```python
from build123d import *

# Parameters (mm, degrees)
CYLINDER009_R     = 0.8
CYLINDER009_DEPTH = 20
CYLINDER010_R     = 0.8
CYLINDER010_DEPTH = 20
CYLINDER011_R     = 0.8
CYLINDER011_DEPTH = 20
CYLINDER008_R     = 0.8
CYLINDER008_DEPTH = 20
CYLINDER005_R     = 0.34
CYLINDER005_DEPTH = 100
CYLINDER006_R     = 0.34
CYLINDER006_DEPTH = 100
CYLINDER007_R     = 0.34
CYLINDER007_DEPTH = 100
CYLINDER004_R     = 0.34
CYLINDER004_DEPTH = 100
CYLINDER002_R     = 4.6
CYLINDER002_DEPTH = 0.5
CYLINDER003_R     = 4.6
CYLINDER003_DEPTH = 0.5
BOX008_W          = 18
BOX008_H          = 9.2
BOX008_DEPTH      = 0.5
BOX004_W          = 40
BOX004_H          = 1
BOX004_DEPTH      = 2.5
CYLINDER001_R     = 2
CYLINDER001_DEPTH = 20
BOX002_W          = 40
BOX002_H          = 42
BOX002_DEPTH      = 6
BOX001_W          = 42
BOX001_H          = 44
BOX001_DEPTH      = 7
BOX003_W          = 40
BOX003_H          = 1
BOX003_DEPTH      = 2.5


with BuildPart() as zylinder009:
    # Cylinder009 → Cylinder009 (new body)
    with BuildSketch(Plane(origin=(2.5, 2.5, -10), x_dir=(1, 0, 0), z_dir=(0, 0, 1))):
        Circle(CYLINDER009_R)
    extrude(amount=CYLINDER009_DEPTH)


with BuildPart() as zylinder010:
    # Cylinder010 → Cylinder010 (new body)
    with BuildSketch(Plane(origin=(37.5, 39.5, -10), x_dir=(1, 0, 0), z_dir=(0, 0, 1))):
        Circle(CYLINDER010_R)
    extrude(amount=CYLINDER010_DEPTH)


with BuildPart() as zylinder011:
    # Cylinder011 → Cylinder011 (new body)
    with BuildSketch(Plane(origin=(2.5, 39.5, -10), x_dir=(1, 0, 0), z_dir=(0, 0, 1))):
        Circle(CYLINDER011_R)
    extrude(amount=CYLINDER011_DEPTH)


with BuildPart() as compound005:
    # Cylinder008 → Cylinder008 (new body)
    with BuildSketch(Plane(origin=(37.5, 2.5, -10), x_dir=(1, 0, 0), z_dir=(0, 0, 1))):
        Circle(CYLINDER008_R)
    extrude(amount=CYLINDER008_DEPTH)

    # Compound005: union Zylinder009, Zylinder010, Zylinder011
    add(zylinder009.part)
    add(zylinder010.part)
    add(zylinder011.part)


with BuildPart() as zylinder005:
    # Cylinder005 → Cylinder005 (new body)
    with BuildSketch(Plane(origin=(18, 28, -50), x_dir=(1, 0, 0), z_dir=(0, 0, 1))):
        Circle(CYLINDER005_R)
    extrude(amount=CYLINDER005_DEPTH)


with BuildPart() as zylinder006:
    # Cylinder006 → Cylinder006 (new body)
    with BuildSketch(Plane(origin=(36, 14.5, -50), x_dir=(1, 0, 0), z_dir=(0, 0, 1))):
        Circle(CYLINDER006_R)
    extrude(amount=CYLINDER006_DEPTH)


with BuildPart() as zylinder007:
    # Cylinder007 → Cylinder007 (new body)
    with BuildSketch(Plane(origin=(36, 27.5, -50), x_dir=(1, 0, 0), z_dir=(0, 0, 1))):
        Circle(CYLINDER007_R)
    extrude(amount=CYLINDER007_DEPTH)


with BuildPart() as m1tapholes:
    # Cylinder004 → Cylinder004 (new body)
    with BuildSketch(Plane(origin=(18, 14, -50), x_dir=(1, 0, 0), z_dir=(0, 0, 1))):
        Circle(CYLINDER004_R)
    extrude(amount=CYLINDER004_DEPTH)

    # Compound002: union Zylinder005, Zylinder006, Zylinder007
    add(zylinder005.part)
    add(zylinder006.part)
    add(zylinder007.part)


with BuildPart() as zylinder002:
    # Cylinder002 → Cylinder002 (new body)
    with BuildSketch(Plane(origin=(27.75, 21, -4.4), x_dir=(1, 0, 0), z_dir=(0, 0, 1))):
        Circle(CYLINDER002_R)
    extrude(amount=CYLINDER002_DEPTH)


with BuildPart() as zylinder003:
    # Cylinder003 → Cylinder003 (new body)
    with BuildSketch(Plane(origin=(27.75, 21, -4.4), x_dir=(1, 0, 0), z_dir=(0, 0, 1))):
        Circle(CYLINDER003_R)
    extrude(amount=CYLINDER003_DEPTH)


with BuildPart() as fusion002:
    # Box008 → Box008 (new body)
    with BuildSketch(Plane(origin=(27.5, 16.4, -4.4), x_dir=(1, 0, 0), z_dir=(0, 0, 1))):
        with Locations((9, 4.6)):
            Rectangle(BOX008_W, BOX008_H)
    extrude(amount=BOX008_DEPTH)

    # Fusion002: union Zylinder002, Zylinder003
    add(zylinder002.part)
    add(zylinder003.part)


with BuildPart() as fusion002_1:
    # Fusion002 placement: moved
    add(fusion002.part.moved(Location((2.3, 0, 0))))


with BuildPart() as obj1:
    # Box004 → Box004 (new body)
    with BuildSketch(Plane(origin=(0, 41, -3.4), x_dir=(1, 0, 0), z_dir=(0, 0, 1))):
        with Locations((20, 0.5)):
            Rectangle(BOX004_W, BOX004_H)
    extrude(amount=BOX004_DEPTH)


with BuildPart() as zylinder001:
    # Cylinder001 → Cylinder001 (new body)
    with BuildSketch(Plane(origin=(30, 21, -10), x_dir=(1, 0, 0), z_dir=(0, 0, 1))):
        Circle(CYLINDER001_R)
    extrude(amount=CYLINDER001_DEPTH)


with BuildPart() as obj2:
    # Box002 → Box002 (new body)
    with BuildSketch(Plane.XY.offset(-3.4)):
        with Locations((20, 21)):
            Rectangle(BOX002_W, BOX002_H)
    extrude(amount=BOX002_DEPTH)


with BuildPart() as cut002:
    # Box001 → Box001 (new body)
    with BuildSketch(Plane(origin=(-1, -1, -4.4), x_dir=(1, 0, 0), z_dir=(0, 0, 1))):
        with Locations((21, 22)):
            Rectangle(BOX001_W, BOX001_H)
    extrude(amount=BOX001_DEPTH)

    # Cut001: cut obj2
    add(obj2.part, mode=Mode.SUBTRACT)

    # Cut002: cut Zylinder001
    add(zylinder001.part, mode=Mode.SUBTRACT)


with BuildPart() as upperpart:
    # Box003 → Box003 (new body)
    with BuildSketch(Plane.XY.offset(-3.4)):
        with Locations((20, 0.5)):
            Rectangle(BOX003_W, BOX003_H)
    extrude(amount=BOX003_DEPTH)

    # Fusion: union obj1, Cut002
    add(obj1.part)
    add(cut002.part)

    # Cut004: cut Fusion002
    add(fusion002_1.part, mode=Mode.SUBTRACT)

    # Cut005: cut M1TapHoles
    add(m1tapholes.part, mode=Mode.SUBTRACT)

    # Cut007: cut Compound005
    add(compound005.part, mode=Mode.SUBTRACT)


solid = upperpart.part
```
The listing builds one solid part. Answer for the finished solid, in the listing's coordinates (mm). A direction names the side the tool comes from. Round coordinates to 2 decimals unless told otherwise and drop trailing zeros. Loops run counter-clockwise (first coordinate to the right, second up) from the corner with the lowest first, then second, coordinate; pieces in that order, holes last.
Q1. Section C-C, the plane z = 1 is taken. Determine the outline of the cut face in (x, y), then the cut area to 3 significant figures.
Q2. Section D-D, the plane y = 21 is taken. Determine the outline of the cut face in (x, z).
Q3. Section A-A, the plane x = 2.5 is taken. Determine the outline of the cut face in (y, z), then the cut area to 3 significant figures.
Q4. Given pin 1 Ø4 at (x, y) = (9.5, 8) entering from +Z; pin 2 Ø0.5 at (x, y) = (20, 0.5) entering from +Z; pin 3 Ø3 at (x, y) = (31, 20) entering from -Z, each flat-ended and moving along its own axis, determine where each tip first touches the part or whether it passes through.
Q5. For a pull along Y with two mould halves and no side action, classify faces 1 (the face through (-0.3, 21.1, 2.6)), 2 (the face through (33, 21, -3.9)), 3 (the face through (20, -1, -1)), 4 (the face through (20, 0, 1)) as released by +Y, released by -Y, zero draft, split by the parting line, or undercut.
Q6. Which of the six approach directions +Z, -Z, +X, -X, +Y, -Y give full straight-line access (tool end or side, diameter ignored) to faces 5 (the face through (38.263, 2.74, -3.907)), 6 (the face through (19.7, 0.5, -0.9))?
Q7. Find the intervals of material crossed by line 1 (Y direction, x = 2.5, z = -3.65); line 2 (Y direction, x = 18, z = -4.15); line 3 (X direction, y = 9.5, z = 0), in increasing order.
Q8. Section B-B, the plane y = 2.5 is taken. Determine the outline of the cut face in (x, z).
Completed:
1. outline: (-1, -1) - (41, -1) - (41, 43) - (-1, 43) - close; hole (0, 0) - (40, 0) - (40, 42) - (0, 42) - close
1. area: 168 mm2
2. outline: (-1, -4.4) - (25.45, -4.4) - (25.45, -3.9) - (28, -3.9) - (28, -3.4) - (0, -3.4) - (0, 2.6) - (-1, 2.6) - close; (32, -3.9) - (41, -3.9) - (41, 2.6) - (40, 2.6) - (40, -3.4) - (32, -3.4) - close
3. outline: (-1, -4.4) - (1.7, -4.4) - (1.7, -3.4) - (1, -3.4) - (1, -0.9) - (0, -0.9) - (0, 2.6) - (-1, 2.6) - close; (3.3, -4.4) - (38.7, -4.4) - (38.7, -3.4) - (3.3, -3.4) - close; (40.3, -4.4) - (43, -4.4) - (43, 2.6) - (42, 2.6) - (42, -0.9) - (41, -0.9) - (41, -3.4) - (40.3, -3.4) - close
3. area: 57.8 mm2
4. pin 1: stops at z = -3.4
4. pin 2: stops at z = -0.9
4. pin 3: stops at z = -3.9
5. face 1: zero draft
5. face 2: undercut
5. face 3: released by -Y
5. face 4: undercut
6. face 5: +Z, -Z
6. face 6: +Z
7. line 1: y = -1 to 1.7, 3.3 to 38.7, 40.3 to 43
7. line 2: y = -1 to 13.66, 14.34 to 27.66, 28.34 to 43
7. line 3: x = -1 to 0, 40 to 41
8. outline: (-1, -4.4) - (1.7, -4.4) - (1.7, -3.4) - (0, -3.4) - (0, 2.6) - (-1, 2.6) - close; (3.3, -4.4) - (36.7, -4.4) - (36.7, -3.4) - (3.3, -3.4) - close; (38.3, -4.4) - (41, -4.4) - (41, 2.6) - (40, 2.6) - (40, -3.4) - (38.3, -3.4) - close
